```python
from build123d import *

# Parameters (mm, degrees)
F0_W     = 78
F0_H     = 93
F1_DEPTH = 163
F2_T     = -2.5
F3_DEPTH = 2.5
F4_DEPTH = 2.5
F5_DEPTH = 25


with BuildPart() as f1:
    # F0 (on Right) → F1 (new body)
    with BuildSketch(Plane.YZ):
        with Locations((-119.8926544255, -26.4388019443)):
            Rectangle(F0_W, F0_H)
    extrude(amount=F1_DEPTH)

    # F2
    f2_openings = [f1.faces().sort_by_distance(p)[0] for p in [
        (81.5, -119.892654, 20.061198),
    ]]
    offset(amount=F2_T, openings=f2_openings)

    # F3 (add): a face of the model
    f3_faces = [f1.faces().sort_by_distance(p)[0] for p in [
        (81.5, -158.8926544255, -26.4388019443),
    ]]
    extrude(f3_faces, amount=-F3_DEPTH)

    # F4 (cut): a face of the model
    f4_faces = [f1.faces().sort_by_distance(p)[0] for p in [
        (81.5, -158.8926544255, -26.4388019443),
    ]]
    extrude(f4_faces, amount=-F4_DEPTH, mode=Mode.SUBTRACT)

    # F5 (cut): a face of the model
    f5_faces = [f1.faces().sort_by_distance(p)[0] for p in [
        (160.5, -119.8926544255, -25.1888019443),
    ]]
    extrude(f5_faces, amount=-F5_DEPTH, mode=Mode.SUBTRACT)


solid = f1.part
```
Here's how the part is built. I have some questions about the finished solid (model axes, mm). A direction names the side the tool comes from. Give positions to 0.01 mm unless a question says otherwise; leave off trailing zeros. Loops run counter-clockwise (first coordinate to the right, second up) from the corner with the lowest first, then second, coordinate; pieces in that order, holes last. Notation, with made-up numbers: M 41,24.5 L 89,24.5 A21 cw 89,60.5 Z; hole C -5.5,54 d5. An arc over 180 degrees is marked long. Use one line per item in the form item = value. Start each with the question number.
Q1. Which directions (+Z, -Z, +X, -X, +Y, -Y) give clear straight access to the entire face, cutting with the end or side of a thin tool? Please do faces 1 (the flat face through (82, -83.393, -26)), 2 (the flat face through (163, -82, -47)).
Q2. If we section it at A-A (y = -136): Write out the boundary of the cut face in (x, z).
Q3. I need wall thicknesses on line 1 along Z through (x, y) = (34, -102.5); line 2 along Y through (x, z) = (22.5, -32.5); line 3 along X through (y, z) = (-107.5, -65.5). Which ranges of each line are inside material? Lowest first, please.
Q4. If we section it at B-B (x = 120): Write out the boundary of the cut face in (y, z), then the cut area to 3 significant figures.
Q5. Will these pins go through, and if not, where does the flat tip stop? pin 1 Ø12 at (x, y) = (43, -116.5) entering from +Z; pin 2 Ø1.5 at (x, z) = (70, -59.5) entering from -Y.
Taken from the geometry:
q1.face_1 = +Z, +X, -Y
q1.face_2 = +Z, -Z, +X, +Y, -Y
q2.outline = M 0,-72.94 L 163,-72.94 L 163,-70.44 L 2.5,-70.44 L 2.5,20.06 L 0,20.06 Z
q3.line_1 = -72.94 to -70.44
q3.line_2 = -83.39 to -80.89
q3.line_3 = 0 to 2.5
q4.outline = M -156.39,-72.94 L -80.89,-72.94 L -80.89,20.06 L -83.39,20.06 L -83.39,-70.44 L -156.39,-70.44 Z
q4.area = 415 mm^2
q5.pin_1 = -70.44
q5.pin_2 = -83.39
